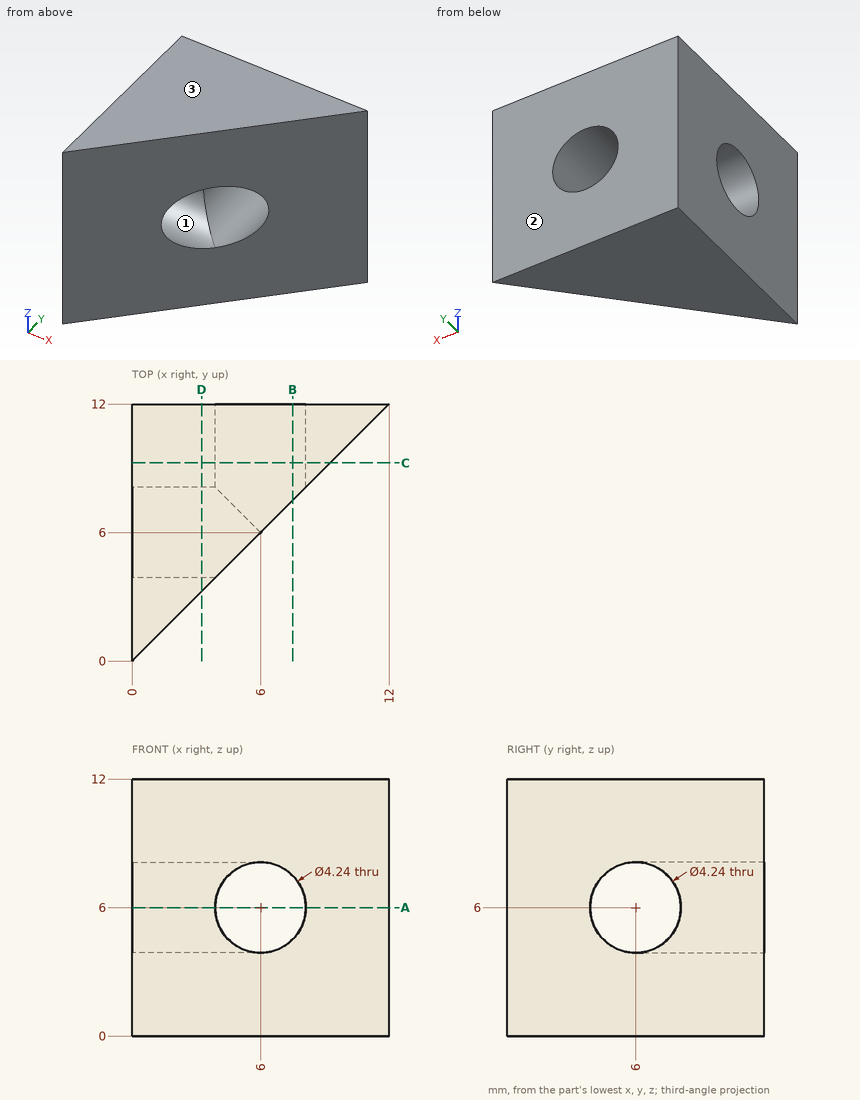
Source: three-view drawing plus pictorial views. Frame: mm from the lowest corner of the part. Round coordinates to 2 decimals unless told otherwise and drop trailing zeros. Order: outer loops, then holes, each group sorted by start corner. A loop starts at its lowest first (then second) coordinate and runs counter-clockwise, first axis right, second up. Notation, with made-up numbers: (-10, 78.5) -> (12, 78.5) arc R11 cw to (12, 93.5) -> close; hole circle Ø11 at (-33.5, 63.5). An arc over 180 degrees is marked (long way). Use one line per item in the form item = value.
(1) Section D-D on x = 3.25. Return loops of the section in (y, z), and give its area (3 significant figures).
Results list:
outline = (3.25, 0) -> (12, 0) -> (12, 12) -> (3.25, 12) -> close; hole circle Ø4.24 at (6, 6)
area = 90.9 mm^2
(2) First-contact query: pin 1 Ø2 at (y, z) = (6.5, 4.5) entering from +X. Flat tip, straight axial feed; report the tip coordinate or a pass-through.
Results list:
pin_1 = 7.5
(3) Draft query along Y for the marked faces 1, 2 and 3. Return one class per face: pulls with the +Y half, pulls with the -Y half, needs draft (parallel to the pull), parting line crosses it, or undercut.
Results list:
face_1 = undercut
face_2 = pulls with the +Y half
face_3 = needs draft
(4) Section A-A on z = 6. Return loops of the section in (x, y), and give its area (3 significant figures).
Results list:
outline = (0, 0) -> (3.88, 3.88) -> (0, 3.88) -> close; (0, 8.12) -> (3.88, 8.12) -> (3.88, 12) -> (0, 12) -> close; (8.12, 8.12) -> (12, 12) -> (8.12, 12) -> close
area = 30.1 mm^2
(5) Section C-C on y = 9.25. Return loops of the section in (x, z), and give its area (3 significant figures).
Results list:
outline = (0, 0) -> (9.25, 0) -> (9.25, 12) -> (0, 12) -> close; hole circle Ø4.24 at (6, 6)
area = 96.9 mm^2
(6) Ray query, probe 1 along Z at (x, y) = (6, 8); probe 2 along Y at (x, z) = (2.85, 6); probe 3 along X at (y, z) = (9.25, 6). Return the intervals inside material, ascending. Write a range as [from, to].
Results list:
probe_1 = [0, 3.88], [8.12, 12]
probe_2 = [2.85, 3.88], [8.12, 12]
probe_3 = [0, 3.88], [8.12, 9.25]
(7) Section B-B on x = 7.5. Return loops of the section in (y, z), and give its area (3 significant figures).
Results list:
outline = (7.5, 0) -> (12, 0) -> (12, 4.5) -> (7.5, 4.5) -> close; (7.5, 7.5) -> (12, 7.5) -> (12, 12) -> (7.5, 12) -> close
area = 40.5 mm^2
